Can you work these out from the model? Positions are in its coordinate system, mm. Face numbers are marked on the shaded views. A direction names the side the tool comes from. Give positions to 0.01 mm unless a question says otherwise; leave off trailing zeros. Write each loop counter-clockwise with the first axis right and the second up, starting at its lowest first coordinate (ties: lowest second). Pieces come first, ordered by that corner, then holes.
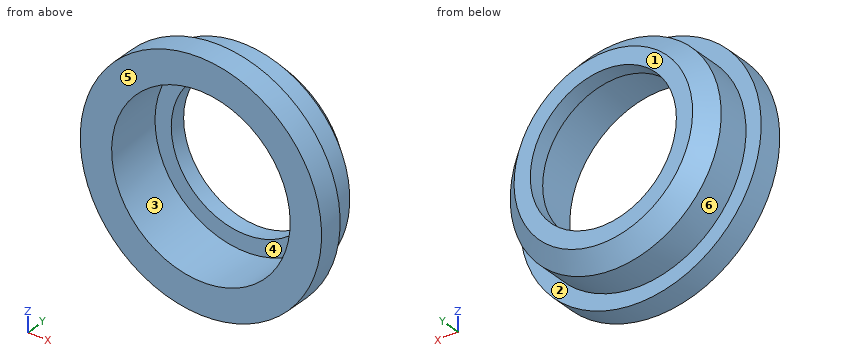
```python
from build123d import *

# Parameters (mm, degrees)
CROQUIS1_R                 = 11
CROQUIS1_R_2               = 2
CROQUIS1_W                 = 30
CROQUIS1_H                 = 3
SALIENTE_EXTRUIR1_DEPTH    = 3
CROQUIS2_R                 = 13
CROQUIS2_R_2               = 11
SALIENTE_EXTRUIR2_DEPTH    = 4
CROQUIS3_R                 = 13
CROQUIS3_R_2               = 9
SALIENTE_EXTRUIR3_DEPTH    = 2
CHAFL_N1_SIZE              = 2
CHAFL_N2_SIZE              = 10
CORTAR_EXTRUIR1_DEPTH      = 10
CORTAR_EXTRUIR1_DEPTH_BACK = 10
CROQUIS4_OUTSIDE_W         = 165.218
CROQUIS4_OUTSIDE_H         = 70.218
CROQUIS4_OUTSIDE_R         = 14.870057098


with BuildPart() as part:
    # Croquis1 → Saliente-Extruir1 (new body)
    with BuildSketch(Plane(origin=(0, 0, 0), x_dir=(1, 0, 0), z_dir=(0, 1, 0))):
        Polygon((65, 10), (70, 15), (70, -15), (65, -10), (65, -20), (-65, -20), (-65, 20), (65, 20), align=None)
        with Locations(Location((-50.129942902, 0, 0), (0, 0, 270))):
            Circle(CROQUIS1_R, mode=Mode.SUBTRACT)
        with Locations(Location((-28.595127909, 0, 0), (0, 0, 270))):
            Circle(CROQUIS1_R_2, mode=Mode.SUBTRACT)
        with Locations(Location((-13.595127909, 0, 0), (0, 0, 270))):
            Circle(CROQUIS1_R_2, mode=Mode.SUBTRACT)
        with Locations(Location((50, 0, 0), (0, 0, 270))):
            Circle(CROQUIS1_R_2, mode=Mode.SUBTRACT)
        with Locations((25, 11)):
            Rectangle(CROQUIS1_W, CROQUIS1_H, mode=Mode.SUBTRACT)
        with Locations((25, -11)):
            Rectangle(CROQUIS1_W, CROQUIS1_H, mode=Mode.SUBTRACT)
    extrude(amount=SALIENTE_EXTRUIR1_DEPTH)

    # Croquis2 → Saliente-Extruir2 (add)
    with BuildSketch(Plane(origin=(0, 3, 0), x_dir=(1, 0, 0), z_dir=(0, 1, 0))):
        with Locations(Location((-50.129942902, 0, 0), (0, 0, 90))):
            Circle(CROQUIS2_R)
        with Locations(Location((-50.129942902, 0, 0), (0, 0, 270))):
            Circle(CROQUIS2_R_2, mode=Mode.SUBTRACT)
    extrude(amount=SALIENTE_EXTRUIR2_DEPTH)

    # Croquis3 → Saliente-Extruir3 (add)
    with BuildSketch(Plane(origin=(0, 7, 0), x_dir=(1, 0, 0), z_dir=(0, 1, 0))):
        with Locations(Location((-50.129942902, 0, 0), (0, 0, 90))):
            Circle(CROQUIS3_R)
        with Locations(Location((-50.129942902, 0, 0), (0, 0, 270))):
            Circle(CROQUIS3_R_2, mode=Mode.SUBTRACT)
    extrude(amount=SALIENTE_EXTRUIR3_DEPTH)

    # Chaflán1
    chafl_n1_edges = [part.edges().sort_by_distance(p)[0] for p in [
        (-50.129942902, 9, 13),
    ]]
    chamfer(chafl_n1_edges, length=CHAFL_N1_SIZE)

    # Chaflán2
    chafl_n2_edges = [part.edges().sort_by_distance(p)[0] for p in [
        (-65, 1.5, 20),
        (-65, 1.5, -20),
    ]]
    chamfer(chafl_n2_edges, length=CHAFL_N2_SIZE)

    # Croquis4 outside → Cortar-Extruir1 (cut, two sides: drawn at the far end of the back side and taken through both)
    with BuildSketch(Plane(origin=(0, 3, 0), x_dir=(1, 0, 0), z_dir=(0, 1, 0)).offset(-CORTAR_EXTRUIR1_DEPTH_BACK)):
        with Locations((2.5, 0)):
            Rectangle(CROQUIS4_OUTSIDE_W, CROQUIS4_OUTSIDE_H)
        with Locations(Location((-50.129942902, 0, 0), (0, 0, 90))):
            Circle(CROQUIS4_OUTSIDE_R, mode=Mode.SUBTRACT)
    extrude(amount=CORTAR_EXTRUIR1_DEPTH + CORTAR_EXTRUIR1_DEPTH_BACK, mode=Mode.SUBTRACT)


solid = part.part
```
1) Suppose I cut it at B-B on y = 6.5. Write out the boundary of the cut face in (x, z), plus the area to 3 significant figures.
Values follow:
outline: circle Ø26 at (-50.13, 0); hole circle Ø22 at (-50.13, 0)
area: 151 mm2
2) If we mould it in two halves opening along Z, with no side actions, what happens to the marked faces 4, 5 and 6? For each: +Z half, -Z half, draft (parallel to the pull), parting line (faces both ways), or undercut.
Values follow:
face 4: undercut
face 5: draft
face 6: parting line
3) Suppose I cut it at A-A on z = 0. Write out the boundary of the cut face in (x, y).
Values follow:
outline: (-65, 0) - (-61.13, 0) - (-61.13, 7) - (-59.13, 7) - (-59.13, 9) - (-61.13, 9) - (-63.13, 7) - (-63.13, 3) - (-65, 3) - close; (-41.13, 7) - (-39.13, 7) - (-39.13, 0) - (-35.26, 0) - (-35.26, 3) - (-37.13, 3) - (-37.13, 7) - (-39.13, 9) - (-41.13, 9) - close
4) Suppose I cut it at C-C on y = 2. Write out the boundary of the cut face in (x, z), plus the area to 3 significant figures.
Values follow:
outline: circle Ø29.74 at (-50.13, 0); hole circle Ø22 at (-50.13, 0)
area: 315 mm2
5) For the marked faces 1, 2 and 3, which set-ups out of +Z, -Z, +X, -X, +Y, -Y let a thin tool reach every point of the face, with its end or its side?
Values follow:
face 1: +Z, -Z, +X, -X, +Y
face 2: +Y
face 3: -Y
6) For pin 1 Ø8 at (x, z) = (-41.5, 3) entering from -Y; pin 2 Ø3 at (y, z) = (8, -6.5) entering from +X; pin 3 Ø13 at (x, z) = (-50.13, 0) entering from +Y; pin 4 Ø1 at (y, z) = (2.5, -2.5) entering from -X, each with a flat end and sliding along its axis, tell me the tip position at first contact or that it passes through.
Values follow:
pin 1: stops at y = 0
pin 2: stops at x = -38.3
pin 3: passes through
pin 4: stops at x = -64.86
7) Please list where these lines run through material, in increasing order: L1, parallel to X at y = 3.75, z = 0.25; L2, parallel to X at y = 1.75, z = 0; L3, parallel to Y at x = -40, z = -2.75.
Values follow:
L1: x = -63.13 to -61.13, -39.13 to -37.13
L2: x = -65 to -61.13, -39.13 to -35.26
L3: y = 7 to 9
